Geometry: final body of the model. Coordinates: model frame, mm. Give positions to 0.01 mm unless a question says otherwise; leave off trailing zeros. Loops run counter-clockwise (first coordinate to the right, second up) from the corner with the lowest first, then second, coordinate; pieces in that order, holes last.
```python
from build123d import *

# Parameters (mm, degrees)
BOSS_EXTRUDE1_DEPTH = 6.35
SKETCH2_R           = 3.175
CUT_EXTRUDE1_DEPTH  = 18.415


with BuildPart() as part:
    # Sketch1 → Boss-Extrude1 (new body)
    with BuildSketch(Plane.XY):
        with BuildLine():
            Line((-27.94, 70.104), (-37.465, 70.104))
            Line((-37.465, 70.104), (-63.5, -31.496))
            Line((-63.5, -31.496), (-63.5, -56.896))
            Line((-63.5, -56.896), (63.5, -56.896))
            Line((63.5, -56.896), (63.5, -31.496))
            Line((63.5, -31.496), (37.465, 70.104))
            Line((37.465, 70.104), (27.94, 70.104))
            ThreePointArc((27.94, 70.104), (0, 42.164), (-27.94, 70.104))
        make_face()
        Polygon((53.667246667, -31.496), (6.6504394, -31.496), (28.29998163, 38.06486673), (32.43650344, 51.355680886), align=None, mode=Mode.SUBTRACT)
        Polygon((-32.43650344, 51.355680886), (-53.667246667, -31.496), (-6.6504394, -31.496), (-28.29998163, 38.06486673), align=None, mode=Mode.SUBTRACT)
        with BuildLine():
            Line((0, -31.496), (22.236848418, 39.951905588))
            ThreePointArc((22.236848418, 39.951905588), (0, 32.639), (-22.236848418, 39.951905588))
            Line((-22.236848418, 39.951905588), (0, -31.496))
        make_face(mode=Mode.SUBTRACT)
    extrude(amount=BOSS_EXTRUDE1_DEPTH)

    # Sketch2 → Cut-Extrude1 (cut)
    with BuildSketch(Plane.XY.offset(6.35)):
        with Locations((-25.4, -44.196)):
            Circle(SKETCH2_R)
        with Locations((25.4, -44.196)):
            Circle(SKETCH2_R)
    extrude(amount=-CUT_EXTRUDE1_DEPTH, mode=Mode.SUBTRACT)


solid = part.part
```
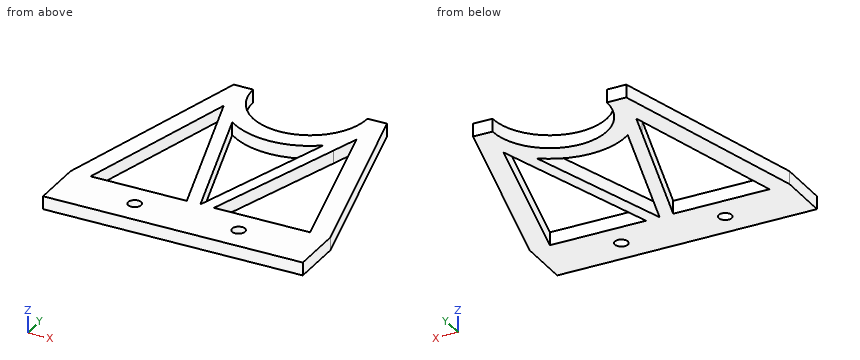
Q1. Material intervals for probe 1 along X at (y, z) = (19, 3.25); probe 2 along X at (y, z) = (-20, 5.5); probe 3 along X at (y, z) = (-43, 4.75), sorted ascending.
Q2. Section query B-B, the plane x = 44. Return loops of the section in (y, z), and give its area (3 significant figures).
Q3. Section query D-D, the plane x = 13. Return loops of the section in (y, z), and give its area (3 significant figures).
Q4. Section query C-C, the plane y = 58. Return loops of the section in (x, z).
Q5. Pin query (flat end, axial travel): pin 1 Ø1 at (y, z) = (-29.5, 5) entering from +X. Return the tip coordinate at first contact, or that it passes through.
Q6. Section query A-A, the plane x = -25.4. Return loops of the section in (y, z), and give its area (3 significant figures).
Resolved:
1. probe 1: x = -50.56 to -40.73, -22.37 to -15.72, 15.72 to 22.37, 40.73 to 50.56
1. probe 2: x = -60.55 to -50.72, -10.23 to -3.58, 3.58 to 10.23, 50.72 to 60.55
1. probe 3: x = -63.5 to -28.34, -22.46 to 22.46, 28.34 to 63.5
2. outline: (-56.9, 0) - (-31.5, 0) - (-31.5, 6.35) - (-56.9, 6.35) - close; (6.23, 0) - (44.6, 0) - (44.6, 6.35) - (6.23, 6.35) - close
2. area: 405 mm2
3. outline: (-56.9, 0) - (-31.5, 0) - (-31.5, 6.35) - (-56.9, 6.35) - close; (-11.09, 0) - (10.27, 0) - (10.27, 6.35) - (-11.09, 6.35) - close; (34.97, 0) - (45.37, 0) - (45.37, 6.35) - (34.97, 6.35) - close
3. area: 363 mm2
4. outline: (-40.57, 0) - (-25.18, 0) - (-25.18, 6.35) - (-40.57, 6.35) - close; (25.18, 0) - (40.57, 0) - (40.57, 6.35) - (25.18, 6.35) - close
5. pin 1: stops at x = 63.12
6. outline: (-56.9, 0) - (-47.37, 0) - (-47.37, 6.35) - (-56.9, 6.35) - close; (-41.02, 0) - (-31.5, 0) - (-31.5, 6.35) - (-41.02, 6.35) - close; (28.75, 0) - (58.46, 0) - (58.46, 6.35) - (28.75, 6.35) - close
6. area: 310 mm2
